Build history of the part. All positions in model axes, mm. Face numbers are marked on the shaded views. A direction names the side the tool comes from. Round coordinates to 2 decimals unless told otherwise and drop trailing zeros. Loops run counter-clockwise (first coordinate to the right, second up) from the corner with the lowest first, then second, coordinate; pieces in that order, holes last. Notation, with made-up numbers: (78.5, 32.25) -> (96.5, 32.25) arc R20 cw to (96.5, 62.25) -> close; hole circle Ø5 at (85, 60). An arc over 180 degrees is marked (long way). Put each result on its own line as item: value. Start each with the question number.
Item 1: Tool access for the marked faces 1 and 2: list every direction of +Z, -Z, +X, -X, +Y, -Y with a clear straight run to the whole face (end or side of a thin tool).
Item 2: Cut at B-B, the plane y = 0.6. Count the separate pieces of the cut face and the enclosed holes in it, plus the area to 3 significant figures.
Item 3: Cut at A-A, the plane x = 3. List the corners of the cut face in (y, z), plus the area to 3 significant figures.
Item 4: Flat gauge pins, fed straight in: pin 1 Ø1.5 at (x, y) = (-9, -2) entering from -Z; pin 2 Ø3.5 at (x, z) = (24, 3.5) entering from -Y; pin 3 Ø1.5 at (y, z) = (-2.5, -5.5) entering from -X; pin 4 Ø1.8 at (x, y) = (-9, -2.5) entering from -Z. Where does each tip first touch, or does it go through?
Item 5: Drill centre lines: probe 1 along X at (y, z) = (0.9, -5); probe 2 along X at (y, z) = (2.75, 0); probe 3 along Y at (x, z) = (19, -5.5). Where is each one in solid material? Low to high. Write a range as [from, to].
Item 6: Pull direction X, two halves, no side cores. Call the marked faces 3, 4 and 5: +X half, -X half, draft (parallel to the pull), parting line (faces both ways), or undercut.
```python
from build123d import *

# Parameters (mm, degrees)
SKETCH_1_W          = 63
SKETCH_1_H          = 15
SKETCH_1_R          = 1.1
SKETCH_1_R_2        = 1.5
SKETCH_1_R_3        = 2.5
EXTRUDE_1_DEPTH     = 2
SKETCH_2_R          = 1.4
EXTRUDE_2_DEPTH     = 2
SKETCH_3_R          = 3
CUT_EXTRUDE_1_DEPTH = 1.5
SKETCH_4_W          = 46
SKETCH_4_H          = 1.5
EXTRUDE_3_DEPTH     = 5
SKETCH_2_3_R        = 0.95
CUT_EXTRUDE_2_DEPTH = 1.5
CUT_EXTRUDE_3_DEPTH = 0.25
SKETCH_1_7_W        = 15
SKETCH_1_7_H        = 15
SKETCH_1_7_R        = 1.5
SKETCH_1_7_R_2      = 1.1
EXTRUDE_4_DEPTH     = 4
SKETCH_1_8_R        = 6
SKETCH_1_8_R_2      = 1.5
SKETCH_1_8_R_3      = 1.1
CUT_EXTRUDE_4_DEPTH = 2
CUT_EXTRUDE_5_DEPTH = 15


with BuildPart() as part:
    # 草图1 → 凸台-拉伸1 (new body)
    with BuildSketch(Plane(origin=(0, 0, 0), x_dir=(1, 0, 0), z_dir=(0, 1, 0))):
        Rectangle(SKETCH_1_W, SKETCH_1_H)
        with Locations(Location((-12.830127019, -2.5, 0), (0, 0, 270))):
            Circle(SKETCH_1_R, mode=Mode.SUBTRACT)
        with Locations(Location((3, 0, 0), (0, 0, 270))):
            Circle(SKETCH_1_R, mode=Mode.SUBTRACT)
        with Locations(Location((-8.5, 0, 0), (0, 0, 270))):
            Circle(SKETCH_1_R_2, mode=Mode.SUBTRACT)
        with Locations(Location((-4.169872981, 2.5, 0), (0, 0, 270))):
            Circle(SKETCH_1_R, mode=Mode.SUBTRACT)
        with Locations(Location((8, 0, 0), (0, 0, 270))):
            Circle(SKETCH_1_R_3, mode=Mode.SUBTRACT)
        with Locations(Location((13, 0, 0), (0, 0, 270))):
            Circle(SKETCH_1_R, mode=Mode.SUBTRACT)
        with Locations(Location((8, 5, 0), (0, 0, 270))):
            Circle(SKETCH_1_R, mode=Mode.SUBTRACT)
        with Locations(Location((24, 3.5, 0), (0, 0, 270))):
            Circle(SKETCH_1_R, mode=Mode.SUBTRACT)
        with Locations(Location((24, -3.5, 0), (0, 0, 270))):
            Circle(SKETCH_1_R, mode=Mode.SUBTRACT)
        with Locations(Location((20.5, 0, 0), (0, 0, 270))):
            Circle(SKETCH_1_R, mode=Mode.SUBTRACT)
        with Locations(Location((24, 0, 0), (0, 0, 270))):
            Circle(SKETCH_1_R_2, mode=Mode.SUBTRACT)
        with Locations(Location((27.5, 0, 0), (0, 0, 270))):
            Circle(SKETCH_1_R, mode=Mode.SUBTRACT)
    extrude(amount=EXTRUDE_1_DEPTH)

    # 草图2 → 凸台-拉伸2 (add)
    with BuildSketch(Plane.XY.offset(7.5)):
        with Locations(Location((-23.5, 0.6, 0), (0, 0, 205.376933525))):
            Circle(SKETCH_2_R)
        with Locations(Location((-8.5, 0.6, 0), (0, 0, 205.376933525))):
            Circle(SKETCH_2_R)
        with Locations(Location((6.5, 0.6, 0), (0, 0, 205.376933525))):
            Circle(SKETCH_2_R)
    extrude(amount=EXTRUDE_2_DEPTH)

    # 草图3 → 切除-拉伸1 (cut)
    with BuildSketch(Plane.XZ):
        with Locations(Location((-8.5, 0, 0), (0, 0, 270))):
            Circle(SKETCH_3_R)
    extrude(amount=-CUT_EXTRUDE_1_DEPTH, mode=Mode.SUBTRACT)

    # 草图4 → 凸台-拉伸3 (add)
    with BuildSketch(Plane.XZ):
        with Locations((-8.5, 6.75)):
            Rectangle(SKETCH_4_W, SKETCH_4_H)
    extrude(amount=EXTRUDE_3_DEPTH)

    # 草图2<3> → 切除-拉伸2 (cut)
    with BuildSketch(Plane.XY.offset(7.5)):
        with Locations((-23.5, -3.4)):
            Circle(SKETCH_2_3_R)
        with Locations((-8.5, -3.4)):
            Circle(SKETCH_2_3_R)
        with Locations((6.5, -3.4)):
            Circle(SKETCH_2_3_R)
    extrude(amount=-CUT_EXTRUDE_2_DEPTH, mode=Mode.SUBTRACT)

    # 草图5 → 切除-拉伸3 (cut)
    with BuildSketch(Plane(origin=(0, 0, 6), x_dir=(-1, 0, 0), z_dir=(0, 0, -1))):
        Polygon((22.403034489, -1.5), (24.596965511, -1.5), (25.693931023, -3.4), (24.596965511, -5.3), (22.403034489, -5.3), (21.306068977, -3.4), align=None)
        Polygon((6.306068977, -3.4), (7.403034489, -1.5), (9.596965511, -1.5), (10.693931023, -3.4), (9.596965511, -5.3), (7.403034489, -5.3), align=None)
        Polygon((-8.693931023, -3.4), (-7.596965511, -1.5), (-5.403034489, -1.5), (-4.306068977, -3.4), (-5.403034489, -5.3), (-7.596965511, -5.3), align=None)
    extrude(amount=-CUT_EXTRUDE_3_DEPTH, mode=Mode.SUBTRACT)

    # 草图1<7> → 凸台-拉伸4 (add)
    with BuildSketch(Plane(origin=(0, 0, 0), x_dir=(1, 0, 0), z_dir=(0, 1, 0))):
        with Locations((24, 0)):
            Rectangle(SKETCH_1_7_W, SKETCH_1_7_H)
        with Locations(Location((24, 0, 0), (0, 0, 270))):
            Circle(SKETCH_1_7_R, mode=Mode.SUBTRACT)
        with Locations(Location((27.5, 0, 0), (0, 0, 270))):
            Circle(SKETCH_1_7_R_2, mode=Mode.SUBTRACT)
        with Locations(Location((24, -3.5, 0), (0, 0, 270))):
            Circle(SKETCH_1_7_R_2, mode=Mode.SUBTRACT)
        with Locations(Location((20.5, 0, 0), (0, 0, 270))):
            Circle(SKETCH_1_7_R_2, mode=Mode.SUBTRACT)
        with Locations(Location((24, 3.5, 0), (0, 0, 270))):
            Circle(SKETCH_1_7_R_2, mode=Mode.SUBTRACT)
    extrude(amount=EXTRUDE_4_DEPTH)

    # 草图1<8> → 切除-拉伸4 (cut)
    with BuildSketch(Plane(origin=(0, 0, 0), x_dir=(1, 0, 0), z_dir=(0, 1, 0))):
        with Locations(Location((24, 0, 0), (0, 0, 270))):
            Circle(SKETCH_1_8_R)
        with Locations(Location((24, 0, 0), (0, 0, 270))):
            Circle(SKETCH_1_8_R_2, mode=Mode.SUBTRACT)
        with Locations(Location((27.5, 0, 0), (0, 0, 270))):
            Circle(SKETCH_1_8_R_3, mode=Mode.SUBTRACT)
        with Locations(Location((24, -3.5, 0), (0, 0, 270))):
            Circle(SKETCH_1_8_R_3, mode=Mode.SUBTRACT)
        with Locations(Location((20.5, 0, 0), (0, 0, 270))):
            Circle(SKETCH_1_8_R_3, mode=Mode.SUBTRACT)
        with Locations(Location((24, 3.5, 0), (0, 0, 270))):
            Circle(SKETCH_1_8_R_3, mode=Mode.SUBTRACT)
    extrude(amount=CUT_EXTRUDE_4_DEPTH, mode=Mode.SUBTRACT)

    # 草图6 → 切除-拉伸5 (cut)
    with BuildSketch(Plane(origin=(0, 0, -7.5), x_dir=(-1, 0, 0), z_dir=(0, 0, -1))):
        Polygon((-16.5, 2), (-18.5, 4), (-16.5, 4), align=None)
    extrude(amount=-CUT_EXTRUDE_5_DEPTH, mode=Mode.SUBTRACT)


solid = part.part
```
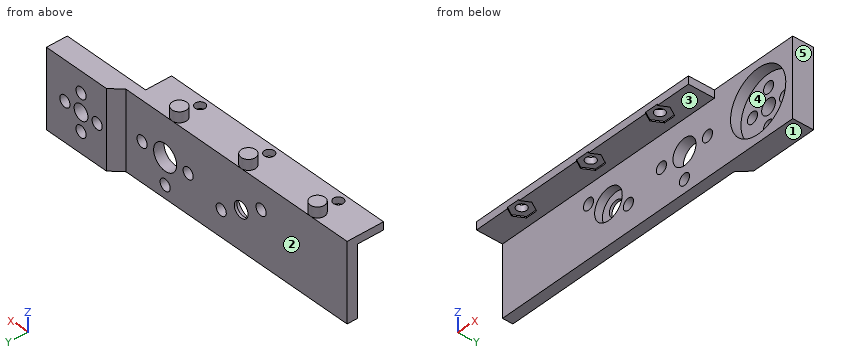
Reply:
1. face 1: -Z, +X, -X, +Y, -Y
1. face 2: +Z, -Z, -X, +Y
2. separate pieces: 1
2. enclosed holes: 8
2. area: 782 mm^2
3. outline: (-5, 6) -> (0, 6) -> (0, 1.1) -> (2, 1.1) -> (2, 7.5) -> (-5, 7.5) -> close; (0, -7.5) -> (2, -7.5) -> (2, -1.1) -> (0, -1.1) -> close
3. area: 33.1 mm^2
4. pin 1: stops at z = 6
4. pin 2: stops at y = 2
4. pin 3: passes through
4. pin 4: stops at z = 6.25
5. probe 1: x = [-31.5, 6.9], [9.1, 20.68], [27.32, 31.5]
5. probe 2: x = [17.25, 19.4], [21.6, 22.5], [25.5, 26.4], [28.6, 31.5]
5. probe 3: y = [0, 4]
6. face 3: draft
6. face 4: undercut
6. face 5: +X half
